Input: part model. Units: mm. Frame: model coordinates. A direction names the side the tool comes from. Round coordinates to 2 decimals unless told otherwise and drop trailing zeros. Loops run counter-clockwise (first coordinate to the right, second up) from the corner with the lowest first, then second, coordinate; pieces in that order, holes last. Notation, with made-up numbers: (-35, 29) - (-19, 29) arc R26 cw to (-19, 65) - close; hole circle Ø7 at (47.5, 78.25). An arc over 180 degrees is marked (long way). Write each question's results on one line, items separated by ' | '.
from build123d import *

# Parameters (mm, degrees)
BOX058_W                  = 0.8
BOX058_H                  = 7.5
BOX058_DEPTH              = 2
CHAMFER029_SIZE2          = 0.8
CHAMFER029_SIZE           = 1
BOX057_W                  = 0.8
BOX057_H                  = 7.5
BOX057_DEPTH              = 2
CHAMFER030_SIZE2          = 0.8
CHAMFER030_SIZE           = 1
BOX061_W                  = 10.2
BOX061_H                  = 0.7
BOX061_DEPTH              = 1
CHAMFER033_SIZE           = 0.3
CYLINDER013_R             = 0.4
CYLINDER013_DEPTH         = 0.5
CYLINDER014_R             = 0.4
CYLINDER014_DEPTH         = 0.5
CYLINDER015_R             = 0.4
CYLINDER015_DEPTH         = 0.7
CYLINDER016_R             = 0.4
CYLINDER016_DEPTH         = 0.7
BOX059_W                  = 0.8
BOX059_H                  = 1.6
BOX059_DEPTH              = 1
BOX060_W                  = 0.8
BOX060_H                  = 1.6
BOX060_DEPTH              = 1
BOX065_W                  = 0.9
BOX065_H                  = 1.8
BOX065_DEPTH              = 1
CHAMFER041_1_SIZE2        = 0.72
CHAMFER041_1_SIZE         = 0.9
CHAMFER041_2_SIZE         = 0.3
BOX064_W                  = 0.9
BOX064_H                  = 1.8
BOX064_DEPTH              = 1
CHAMFER042_1_SIZE2        = 0.72
CHAMFER042_1_SIZE         = 0.9
CHAMFER042_2_SIZE         = 0.3
BOX056_W                  = 10.2
BOX056_H                  = 1
BOX056_DEPTH              = 1.5
CHAMFER028_SIZE2          = 0.9
CHAMFER028_SIZE           = 0.3
FUSION014_PLACEMENT_ANGLE = 12


with BuildPart() as obj1:
    # Box058 → Box058 (new body)
    with BuildSketch(Plane(origin=(-5.1, -6, 0.5), x_dir=(1, 0, 0), z_dir=(0, 0, 1))):
        with Locations((0.4, 3.75)):
            Rectangle(BOX058_W, BOX058_H)
    extrude(amount=BOX058_DEPTH)

    # Chamfer029
    chamfer029_edges = [obj1.edges().sort_by_distance(p)[0] for p in [
        (-4.7, 1.5, 2.5),
    ]]
    chamfer029_side = obj1.faces().sort_by_distance((-4.7, 1.5, 1.5))[0]
    chamfer(chamfer029_edges, length=CHAMFER029_SIZE, length2=CHAMFER029_SIZE2, reference=chamfer029_side)


with BuildPart() as obj2:
    # Box057 → Box057 (new body)
    with BuildSketch(Plane(origin=(4.3, -6, 0.5), x_dir=(1, 0, 0), z_dir=(0, 0, 1))):
        with Locations((0.4, 3.75)):
            Rectangle(BOX057_W, BOX057_H)
    extrude(amount=BOX057_DEPTH)

    # Chamfer030
    chamfer030_edges = [obj2.edges().sort_by_distance(p)[0] for p in [
        (4.7, 1.5, 2.5),
    ]]
    chamfer030_side = obj2.faces().sort_by_distance((4.7, 1.5, 1.5))[0]
    chamfer(chamfer030_edges, length=CHAMFER030_SIZE, length2=CHAMFER030_SIZE2, reference=chamfer030_side)


with BuildPart() as obj3:
    # Box061 → Box061 (new body)
    with BuildSketch(Plane(origin=(-5.1, 3.1, 0.5), x_dir=(1, 0, 0), z_dir=(0, 0, 1))):
        with Locations((5.1, 0.35)):
            Rectangle(BOX061_W, BOX061_H)
    extrude(amount=BOX061_DEPTH)

    # Chamfer033
    chamfer033_edges = [obj3.edges().sort_by_distance(p)[0] for p in [
        (0, 3.8, 0.5),
        (0, 3.8, 1.5),
    ]]
    chamfer(chamfer033_edges, length=CHAMFER033_SIZE)


with BuildPart() as obj4:
    # Cylinder013 → Cylinder013 (new body)
    with BuildSketch(Plane(origin=(-6.5, 3.4, 0.9), x_dir=(0, 0, -1), z_dir=(1, 0, 0))):
        Circle(CYLINDER013_R)
    extrude(amount=CYLINDER013_DEPTH)


with BuildPart() as obj5:
    # Cylinder014 → Cylinder014 (new body)
    with BuildSketch(Plane(origin=(6, 3.4, 0.9), x_dir=(0, 0, -1), z_dir=(1, 0, 0))):
        Circle(CYLINDER014_R)
    extrude(amount=CYLINDER014_DEPTH)


with BuildPart() as obj6:
    # Cylinder015 → Cylinder015 (new body)
    with BuildSketch(Plane(origin=(-5.8, -5.6, 2.1), x_dir=(0, 0, -1), z_dir=(1, 0, 0))):
        Circle(CYLINDER015_R)
    extrude(amount=CYLINDER015_DEPTH)


with BuildPart() as obj7:
    # Cylinder016 → Cylinder016 (new body)
    with BuildSketch(Plane(origin=(5.1, -5.6, 2.1), x_dir=(0, 0, -1), z_dir=(1, 0, 0))):
        Circle(CYLINDER016_R)
    extrude(amount=CYLINDER016_DEPTH)


with BuildPart() as obj8:
    # Box059 → Box059 (new body)
    with BuildSketch(Plane(origin=(-5.1, 1.5, 0.5), x_dir=(1, 0, 0), z_dir=(0, 0, 1))):
        with Locations((0.4, 0.8)):
            Rectangle(BOX059_W, BOX059_H)
    extrude(amount=BOX059_DEPTH)


with BuildPart() as obj9:
    # Box060 → Box060 (new body)
    with BuildSketch(Plane(origin=(4.3, 1.5, 0.5), x_dir=(1, 0, 0), z_dir=(0, 0, 1))):
        with Locations((0.4, 0.8)):
            Rectangle(BOX060_W, BOX060_H)
    extrude(amount=BOX060_DEPTH)


with BuildPart() as obj10:
    # Box065 → Box065 (new body)
    with BuildSketch(Plane(origin=(-6, 2, 0.5), x_dir=(1, 0, 0), z_dir=(0, 0, 1))):
        with Locations((0.45, 0.9)):
            Rectangle(BOX065_W, BOX065_H)
    extrude(amount=BOX065_DEPTH)

    # Chamfer041 1
    chamfer041_1_edges = [obj10.edges().sort_by_distance(p)[0] for p in [
        (-5.55, 2, 1.5),
    ]]
    chamfer041_1_side = obj10.faces().sort_by_distance((-5.55, 2, 1))[0]
    chamfer(chamfer041_1_edges, length=CHAMFER041_1_SIZE, length2=CHAMFER041_1_SIZE2, reference=chamfer041_1_side)

    # Chamfer041 2
    chamfer041_2_edges = [obj10.edges().sort_by_distance(p)[0] for p in [
        (-5.55, 3.8, 0.5),
        (-5.55, 3.8, 1.5),
    ]]
    chamfer(chamfer041_2_edges, length=CHAMFER041_2_SIZE)


with BuildPart() as obj11:
    # Box064 → Box064 (new body)
    with BuildSketch(Plane(origin=(5.1, 2, 0.5), x_dir=(1, 0, 0), z_dir=(0, 0, 1))):
        with Locations((0.45, 0.9)):
            Rectangle(BOX064_W, BOX064_H)
    extrude(amount=BOX064_DEPTH)

    # Chamfer042 1
    chamfer042_1_edges = [obj11.edges().sort_by_distance(p)[0] for p in [
        (5.55, 2, 1.5),
    ]]
    chamfer042_1_side = obj11.faces().sort_by_distance((5.55, 2, 1))[0]
    chamfer(chamfer042_1_edges, length=CHAMFER042_1_SIZE, length2=CHAMFER042_1_SIZE2, reference=chamfer042_1_side)

    # Chamfer042 2
    chamfer042_2_edges = [obj11.edges().sort_by_distance(p)[0] for p in [
        (5.55, 3.8, 0.5),
        (5.55, 3.8, 1.5),
    ]]
    chamfer(chamfer042_2_edges, length=CHAMFER042_2_SIZE)


with BuildPart() as obj12:
    # Box056 → Box056 (new body)
    with BuildSketch(Plane(origin=(-5.1, -7, 1), x_dir=(1, 0, 0), z_dir=(0, 0, 1))):
        with Locations((5.1, 0.5)):
            Rectangle(BOX056_W, BOX056_H)
    extrude(amount=BOX056_DEPTH)

    # Chamfer028
    chamfer028_edges = [obj12.edges().sort_by_distance(p)[0] for p in [
        (0, -7, 2.5),
    ]]
    chamfer028_side = obj12.faces().sort_by_distance((0, -7, 1.75))[0]
    chamfer(chamfer028_edges, length=CHAMFER028_SIZE, length2=CHAMFER028_SIZE2, reference=chamfer028_side)

    # Fusion014: union obj1, obj2, obj3, obj4, obj5, obj6, obj7, obj8, obj9, obj10, obj11
    add(obj1.part)
    add(obj2.part)
    add(obj3.part)
    add(obj4.part)
    add(obj5.part)
    add(obj6.part)
    add(obj7.part)
    add(obj8.part)
    add(obj9.part)
    add(obj10.part)
    add(obj11.part)


with BuildPart() as obj12_1:
    # Fusion014 placement: moved
    add(obj12.part.moved(Location((0, 0, 0.769273))).rotate(Axis((0, 0, 0.769273), (-1, 0, 0)), FUSION014_PLACEMENT_ANGLE))


solid = obj12_1.part
1. Mould query, pull axis X, two halves, no side actions, for faces 6 (the flat face through (-4.3, -1, 3)), 7 (the flat face through (-0.07, -5.91, 4.43)), 8 (the flat face through (5.8, -5, 4)). Classes: pulls with the +X half, pulls with the -X half, needs draft (parallel to the pull), parting line crosses it, or undercut.
Answer:
face 6: undercut | face 7: needs draft | face 8: pulls with the +X half
2. Section query B-B, the plane z = 2.8. Output: boundary loops of the cut face in (x, y).
Answer:
outline: (-5.1, -5.7) - (-4.3, -5.7) - (-4.3, 1.34) - (-5.1, 1.34) - close; (4.3, -5.7) - (5.1, -5.7) - (5.1, 1.34) - (4.3, 1.34) - close
3. Line query: line 1 (X direction, y = 0, z = 2.4); line 2 (Y direction, x = -1, z = 3.4); line 3 (Y direction, x = 4.75, z = 2.65). Output: solid intervals per line, ascending. Write a range as [from, to].
Answer:
line 1: [-5.1, -4.3], [4.3, 5.1] | line 2: [-6.6, -5.57] | line 3: [-5.73, 1.41]
4. Contact query for flat-ended pins moving along their axis: pin 1 (0.6 mm diameter, centred on y = 2.5, z = 1.5, fed in from +X); pin 2 (1.2 mm diameter, centred on y = 0.5, z = 2, fed in from +X); pin 3 (0.9 mm diameter, centred on y = -5, z = 4, fed in from -X); pin 4 (2 mm diameter, centred on x = 2.5, y = 2, fed in from +Z). Output: stop coordinate, or through.
Answer:
pin 1: x = 6 | pin 2: x = 5.1 | pin 3: x = -5.8 | pin 4: through
5. Section query C-C, the plane y = -2. Output: boundary loops of the cut face in (x, z).
Answer:
outline: (-5.1, 1.71) - (-4.3, 1.71) - (-4.3, 3.75) - (-5.1, 3.75) - close; (4.3, 1.71) - (5.1, 1.71) - (5.1, 3.75) - (4.3, 3.75) - close
6. Section query A-A, the plane x = -3.25. Output: boundary loops of the cut face in (y, z), plus the area to 4 significant figures.
Answer:
outline: (-6.64, 3.2) - (-5.66, 2.99) - (-5.35, 4.46) - (-5.45, 4.48) - (-6.39, 4.38) - close; (3.14, 0.61) - (3.53, 0.53) - (3.88, 0.76) - (3.97, 1.15) - (3.74, 1.51) - (3.34, 1.59) - close | area: 1.975 mm^2
7. Set-up query: faces 1 (the flat face through (-0.03, 3.38, 0.56)), 2 (the cylindrical face through (-5.45, -5.21, 4.35)), 3 (the cylindrical face through (5.45, -5.21, 4.35)), 4 (the flat face through (-5.56, 2.53, 1.31)), 5 (the flat face through (5.54, 2.53, 1.31)). Return all of +Z, -Z, +X, -X, +Y, -Y with unobstructed straight access to the full face (end or side cutting, diameter ignored); none if empty.
Answer:
face 1: -Z, +X, -X, -Y | face 2: -X | face 3: +X | face 4: +Z, -X, -Y | face 5: +Z, +X, -Y
